```python
from build123d import *

# Parameters (mm, degrees)
SKIZZE1_W                       = 45
SKIZZE1_H                       = 2.5
AUFSATZ_LINEAR_AUSTRAGEN1_DEPTH = 45
AUFSATZ_LINEAR_AUSTRAGEN2_DEPTH = 22.5
SKIZZE3_R                       = 11.25
SCHNITT_LINEAR_AUSTRAGEN1_DEPTH = 95.007978385
SKIZZE4_R                       = 1.7
SCHNITT_LINEAR_AUSTRAGEN2_DEPTH = 95.007978385
SKIZZE5_R                       = 1.7
SCHNITT_LINEAR_AUSTRAGEN3_DEPTH = 78.942286341


with BuildPart() as part:
    # Skizze1 → Aufsatz-Linear austragen1 (new, symmetric)
    with BuildSketch(Plane.XY):
        with Locations((22.5, 1.25)):
            Rectangle(SKIZZE1_W, SKIZZE1_H)
    extrude(amount=AUFSATZ_LINEAR_AUSTRAGEN1_DEPTH, both=True)

    # Skizze2 → Aufsatz-Linear austragen2 (add, symmetric)
    with BuildSketch(Plane.XY):
        Polygon((0, 0), (-25, 0), (-25, 47.5), (-22.5, 47.5), (-22.5, 2.5), (0, 2.5), align=None)
    extrude(amount=AUFSATZ_LINEAR_AUSTRAGEN2_DEPTH, both=True)

    # Skizze3 → Schnitt-Linear austragen1 (cut, through all)
    with BuildSketch(Plane(origin=(-22.5, 0, 0), x_dir=(0, 0, -1), z_dir=(1, 0, 0))):
        with Locations(Location((0, 25, 0), (0, 0, 90))):
            Circle(SKIZZE3_R)
    extrude(amount=-SCHNITT_LINEAR_AUSTRAGEN1_DEPTH, mode=Mode.SUBTRACT)

    # Skizze4 → Schnitt-Linear austragen2 (cut, through all)
    with BuildSketch(Plane(origin=(-22.5, 0, 0), x_dir=(0, 0, -1), z_dir=(1, 0, 0))):
        with Locations(Location((-9.899494937, 34.899494937, 0), (0, 0, 90))):
            Circle(SKIZZE4_R)
        with Locations(Location((9.899494937, 34.899494937, 0), (0, 0, 270))):
            Circle(SKIZZE4_R)
        with Locations(Location((-9.899494937, 15.100505063, 0), (0, 0, 270))):
            Circle(SKIZZE4_R)
        with Locations(Location((9.899494937, 15.100505063, 0), (0, 0, 90))):
            Circle(SKIZZE4_R)
    extrude(amount=-SCHNITT_LINEAR_AUSTRAGEN2_DEPTH, mode=Mode.SUBTRACT)

    # Skizze5 → Schnitt-Linear austragen3 (cut, through all)
    with BuildSketch(Plane(origin=(0, 2.5, 0), x_dir=(1, 0, 0), z_dir=(0, 1, 0))):
        with Locations(Location((7.5, 37.5, 0), (0, 0, 180))):
            Circle(SKIZZE5_R)
        with Locations(Location((7.5, 30, 0), (0, 0, 180))):
            Circle(SKIZZE5_R)
        with Locations(Location((22.5, 37.5, 0), (0, 0, 180))):
            Circle(SKIZZE5_R)
        with Locations(Location((37.5, 37.5, 0), (0, 0, 180))):
            Circle(SKIZZE5_R)
        with Locations((7.5, -30)):
            Circle(SKIZZE5_R)
        with Locations((37.5, -37.5)):
            Circle(SKIZZE5_R)
        with Locations((22.5, -37.5)):
            Circle(SKIZZE5_R)
        with Locations((7.5, -37.5)):
            Circle(SKIZZE5_R)
    extrude(amount=-SCHNITT_LINEAR_AUSTRAGEN3_DEPTH, mode=Mode.SUBTRACT)


solid = part.part
```
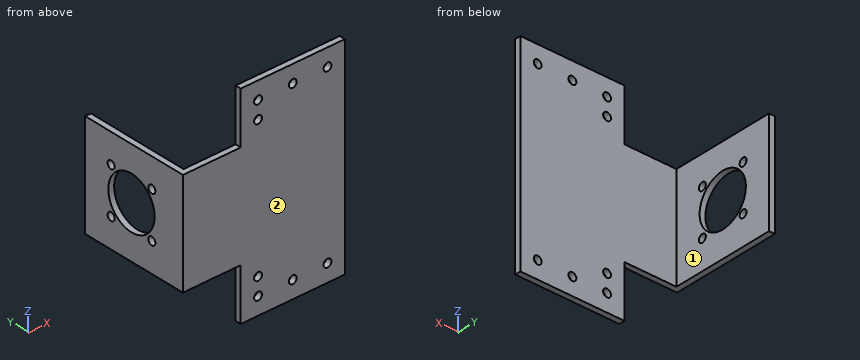
The model under review builds one solid part; all positions refer to its coordinate system, in mm. Face numbers are marked on the shaded views. A direction names the side the tool comes from. Give positions to 0.01 mm unless a question says otherwise; leave off trailing zeros. Write each loop counter-clockwise with the first axis right and the second up, starting at its lowest first coordinate (ties: lowest second). Pieces come first, ordered by that corner, then holes. Notation, with made-up numbers: M 89,73.25 L 108,73.25 A22 cw 108,110.25 Z; hole C 9.25,72 d2. An arc over 180 degrees is marked long. Answer in a Markdown table with one row per item.
Item 1: For line 1 along X through (y, z) = (0.8, 37.5); line 2 along Z through (x, y) = (22.5, 0.5); line 3 along X through (y, z) = (1, 37), list the stretches that pass through material, from the lowest coordinate up.
Check sheet entries:
| item | result |
|---|---|
| line 1 | 0 to 5.8, 9.2 to 20.8, 24.2 to 35.8, 39.2 to 45 |
| line 2 | -45 to -39.2, -35.8 to 35.8, 39.2 to 45 |
| line 3 | 0 to 5.88, 9.12 to 20.88, 24.12 to 35.88, 39.12 to 45 |
Item 2: For P1, Ø2, axis at x = 37.5, z = 37.5, coming from the +Y side; P2, Ø4.5, axis at y = 15.1, z = 9.9, coming from the +X side; P3, Ø1.2, axis at y = 1.5, z = 31, coming from the -X side; P4, Ø4.5, axis at x = 7.5, z = -37.5, coming from the +Y side, all flat-tipped, find the tip position at first contact; note any pin that passes through.
Check sheet entries:
| item | result |
|---|---|
| P1 | through |
| P2 | x = -22.5 |
| P3 | x = 0 |
| P4 | y = 2.5 |
Item 3: Tool access review of the marked faces 1 and 2: name each direction out of +Z, -Z, +X, -X, +Y, -Y from which nothing blocks a thin tool from reaching the whole face with its end or side.
Check sheet entries:
| item | result |
|---|---|
| face 1 | +Z, -Z, +X, +Y |
| face 2 | +Z, -Z, +X, -X, -Y |
Item 4: Add section D-D on y = 15. Give the boundary of the cut face in (x, z).
Check sheet entries:
| item | result |
|---|---|
| outline | M -25,-22.5 L -22.5,-22.5 L -22.5,-11.6 L -25,-11.6 Z; M -25,-8.2 L -22.5,-8.2 L -22.5,-5.15 L -25,-5.15 Z; M -25,5.15 L -22.5,5.15 L -22.5,8.2 L -25,8.2 Z; M -25,11.6 L -22.5,11.6 L -22.5,22.5 L -25,22.5 Z |
Item 5: Add section C-C on z = 30. Give the boundary of the cut face in (x, y), plus the area to 3 significant figures.
Check sheet entries:
| item | result |
|---|---|
| outline | M 0,0 L 5.8,0 L 5.8,2.5 L 0,2.5 Z; M 9.2,0 L 45,0 L 45,2.5 L 9.2,2.5 Z |
| area | 104 mm2 |
Item 6: Add section A-A on x = 7.5. Give the boundary of the cut face in (y, z).
Check sheet entries:
| item | result |
|---|---|
| outline | M 0,-45 L 2.5,-45 L 2.5,-39.2 L 0,-39.2 Z; M 0,-35.8 L 2.5,-35.8 L 2.5,-31.7 L 0,-31.7 Z; M 0,-28.3 L 2.5,-28.3 L 2.5,28.3 L 0,28.3 Z; M 0,31.7 L 2.5,31.7 L 2.5,35.8 L 0,35.8 Z; M 0,39.2 L 2.5,39.2 L 2.5,45 L 0,45 Z |
Item 7: Add section B-B on y = 25. Give the boundary of the cut face in (x, z), plus the area to 4 significant figures.
Check sheet entries:
| item | result |
|---|---|
| outline | M -25,-22.5 L -22.5,-22.5 L -22.5,-11.25 L -25,-11.25 Z; M -25,11.25 L -22.5,11.25 L -22.5,22.5 L -25,22.5 Z |
| area | 56.25 mm2 |
